from build123d import *

# Parameters (mm, degrees)
SKETCH_1_R      = 1.5
SKETCH_1_R_2    = 2.5
EXTRUDE_1_DEPTH = 4


with BuildPart() as part:
    # Sketch 1 → Extrude 1 (new body)
    with BuildSketch(Plane(origin=(0, 0, 0), x_dir=(1, 0, 0), z_dir=(0, 1, 0))):
        Polygon((-21, -21), (21, 21), (57, 21), (57, 13), (-13, -57), (-21, -57), align=None)
        with Locations(Location((53, 17, 0), (0, 0, 270))):
            Circle(SKETCH_1_R, mode=Mode.SUBTRACT)
        with Locations(Location((25, 17, 0), (0, 0, 90))):
            Circle(SKETCH_1_R, mode=Mode.SUBTRACT)
        with Locations(Location((-17, -53, 0), (0, 0, 90))):
            Circle(SKETCH_1_R, mode=Mode.SUBTRACT)
        with Locations(Location((-17, -25, 0), (0, 0, 270))):
            Circle(SKETCH_1_R, mode=Mode.SUBTRACT)
        with Locations(Location((32.960155108, -0.433243174, 0), (0, 0, 270))):
            Circle(SKETCH_1_R_2, mode=Mode.SUBTRACT)
        with Locations(Location((0.433243174, -32.960155108, 0), (0, 0, 90))):
            Circle(SKETCH_1_R_2, mode=Mode.SUBTRACT)
    extrude(amount=EXTRUDE_1_DEPTH)


solid = part.part
The model under review builds one solid part; all positions refer to its coordinate system, in mm. Coordinates: 2 decimals unless noted, no trailing zeros. Order: outer loops, then holes, each group sorted by start corner. A loop starts at its lowest first (then second) coordinate and runs counter-clockwise, first axis right, second up. Notation, with made-up numbers: (72, -23) -> (109, -23) arc R8 ccw to (109, -16) -> close; hole circle Ø8 at (7.5, 9). An arc over 180 degrees is marked (long way). Answer in a Markdown table with one row per item.
(1) Consider section D-D (y = 1.95). Write out the cut boundary in (x, z), plus the area to 3 significant figures.
Answers:
| item | result |
|---|---|
| outline | (-21, 21) -> (21, -21) -> (57, -21) -> (57, -13) -> (-13, 57) -> (-21, 57) -> close; hole circle Ø3 at (-17, 25); hole circle Ø3 at (-17, 53); hole circle Ø5 at (0.43, 32.96); hole circle Ø3 at (25, -17); hole circle Ø5 at (32.96, 0.43); hole circle Ø3 at (53, -17) |
| area | 2,680 mm² |
(2) Insertion check: pin 1 (2 mm diameter, centred on y = 2, z = 19, fed in from +X); pin 2 (1.5 mm diameter, centred on y = 2.5, z = 43, fed in from +X); pin 3 (1 mm diameter, centred on y = 2, z = -7.5, fed in from +X). Each pin has a flat end and moves straight along its axis. Give the tip position at first contact, or say it passes through.
Answers:
| item | result |
|---|---|
| pin 1 | x = 26 |
| pin 2 | x = 1.75 |
| pin 3 | x = 52 |
(3) Consider section C-C (x = -17). Write out the cut boundary in (y, z), plus the area to 3 significant figures.
Answers:
| item | result |
|---|---|
| outline | (0, 17) -> (4, 17) -> (4, 23.5) -> (0, 23.5) -> close; (0, 26.5) -> (4, 26.5) -> (4, 51.5) -> (0, 51.5) -> close; (0, 54.5) -> (4, 54.5) -> (4, 57) -> (0, 57) -> close |
| area | 136 mm² |
(4) Consider section B-B (z = 53). Write out the cut boundary in (x, y).
Answers:
| item | result |
|---|---|
| outline | (-21, 0) -> (-18.5, 0) -> (-18.5, 4) -> (-21, 4) -> close; (-15.5, 0) -> (-9, 0) -> (-9, 4) -> (-15.5, 4) -> close |
(5) Consider section A-A (x = 25). Write out the cut boundary in (y, z).
Answers:
| item | result |
|---|---|
| outline | (0, -21) -> (4, -21) -> (4, -18.5) -> (0, -18.5) -> close; (0, -15.5) -> (4, -15.5) -> (4, 19) -> (0, 19) -> close |
(6) Wall thickness on line 1 along X through (y, z) = (1.9, 25); line 2 along Z through (x, y) = (2, 3.05): over which ranges is each line inside the solid? List them lowest first.
Answers:
| item | result |
|---|---|
| line 1 | -21 to -18.5, -15.5 to 19 |
| line 2 | -2 to 31.01, 34.91 to 42 |
(7) The part is to be moulded in two halves that separate along Z. For faces 1 (the cylindrical face through (-16.93, 1.97, 23.5)), 2 (the flat face through (22, 2, 22)), 3 (the flat face through (10, 4, 9)), say which applies: +Z half, -Z half, draft (parallel to the pull), parting line (faces both ways), or undercut.
Answers:
| item | result |
|---|---|
| face 1 | undercut |
| face 2 | +Z half |
| face 3 | draft |
